Geometry: final body of the model. Coordinates: model frame, mm. A direction names the side the tool comes from. Give positions to 0.01 mm unless a question says otherwise; leave off trailing zeros. Loops run counter-clockwise (first coordinate to the right, second up) from the corner with the lowest first, then second, coordinate; pieces in that order, holes last.
1. Section C-C, the plane x = -10. Output: boundary loops of the cut face in (y, z).
2. Draft query along X for faces 3 (the face through (-6.32, 3.21, 2.81)), 4 (the face through (0, 2, -5)), 5 (the face through (19.4, 2.03, 4.43)), 6 (the face through (-20, 2, 0)). Return one class per face: +X half, -X half, draft (parallel to the pull), parting line (faces both ways), or undercut.
3. Section A-A, the plane z = 0. Output: boundary loops of the cut face in (x, y), then the cut area to 3 significant figures.
4. Section B-B, the plane y = 3. Output: boundary loops of the cut face in (x, z).
5. First-contact query: P1, Ø2, axis at x = -1.5, z = -1, coming from the +Y side. Flat tip, straight axial feed; report the tip coordinate or a pass-through.
6. Access query for faces 1 (the face through (-19.43, 2.03, -4.4)), 2 (the face through (-6.08, 3.21, -2.79)). Directions: +Z, -Z, +X, -X, +Y, -Y. A direction counts if a zero-diameter tool reaches every point of the face in a straight line with its end or side. Return the directions, or none.
7. Material intervals for line 1 along Y through (x, z) = (-14, -0.25); line 2 along Z through (x, y) = (-5, 3.6); line 3 along X through (y, z) = (3.25, 1.5), sorted ascending.
from build123d import *

# Parameters (mm, degrees)
SKETCH_1_W          = 40
SKETCH_1_H          = 10
EXTRUDE_1_DEPTH     = 4
CUT_EXTRUDE_1_DEPTH = 1.6
FILLET_1_R          = 2


with BuildPart() as part:
    # 스케치1 → 보스-돌출1 (new body)
    with BuildSketch(Plane(origin=(0, 0, 0), x_dir=(1, 0, 0), z_dir=(0, 1, 0))):
        Rectangle(SKETCH_1_W, SKETCH_1_H)
    extrude(amount=EXTRUDE_1_DEPTH)

    # 스케치2 → 컷-돌출1 (cut)
    with BuildSketch(Plane(origin=(0, 4, 0), x_dir=(1, 0, 0), z_dir=(0, 1, 0))):
        with BuildLine():
            Line((-14.703333421, -3.5), (2.296666579, -2.1))
            ThreePointArc((2.296666579, -2.1), (4.396666579, 0), (2.296666579, 2.1))
            Line((2.296666579, 2.1), (-14.703333421, 3.5))
            ThreePointArc((-14.703333421, 3.5), (-18.203333421, 0), (-14.703333421, -3.5))
        make_face()
    extrude(amount=-CUT_EXTRUDE_1_DEPTH, mode=Mode.SUBTRACT)

    # 필렛1
    fillet_1_edges = [part.edges().sort_by_distance(p)[0] for p in [
        (20, 2, 5),
        (-20, 2, 5),
        (-20, 2, -5),
        (20, 2, -5),
    ]]
    fillet(fillet_1_edges, radius=FILLET_1_R)


solid = part.part
Answers below:
1. outline: (0, -5) - (4, -5) - (4, -3.11) - (2.4, -3.11) - (2.4, 3.11) - (4, 3.11) - (4, 5) - (0, 5) - close
2. face 3: undercut
2. face 4: draft
2. face 5: +X half
2. face 6: -X half
3. outline: (-20, 0) - (20, 0) - (20, 4) - (4.4, 4) - (4.4, 2.4) - (-18.2, 2.4) - (-18.2, 4) - (-20, 4) - close
3. area: 124 mm2
4. outline: (-20, -3) arc R2 ccw to (-18, -5) - (18, -5) arc R2 ccw to (20, -3) - (20, 3) arc R2 ccw to (18, 5) - (-18, 5) arc R2 ccw to (-20, 3) - close; hole (-14.7, -3.5) - (2.3, -2.1) arc R2.1 ccw to (2.3, 2.1) - (-14.7, 3.5) arc R3.5 ccw to start
5. P1: stops at y = 2.4
6. face 1: -Z, -X, +Y, -Y
6. face 2: +Y
7. line 1: y = 0 to 2.4
7. line 2: z = -5 to -2.7, 2.7 to 5
7. line 3: x = -20 to -17.87, 3.77 to 20
